Check sheet for the modelled part. Datum: model origin and axes. Units: mm. A direction names the side the tool comes from. Give positions to 0.01 mm unless a question says otherwise; leave off trailing zeros. Order: outer loops, then holes, each group sorted by start corner. A loop starts at its lowest first (then second) coordinate and runs counter-clockwise, first axis right, second up. Notation, with made-up numbers: (74, 64) -> (86, 64) arc R16 cw to (86, 86) -> close; hole circle Ø10 at (43.5, 65.25). An arc over 180 degrees is marked (long way). Write each question's results on one line, items separated by ' | '.
from build123d import *

# Parameters (mm, degrees)
SKETCH1_R           = 11.25
SKETCH1_R_2         = 11.05
BOSS_EXTRUDE1_DEPTH = 20
BOSS_EXTRUDE2_DEPTH = 2
SKETCH3_R           = 9.5
BOSS_EXTRUDE3_DEPTH = 18
SKETCH4_W           = 81.5
SKETCH4_H           = 10
CUT_EXTRUDE1_DEPTH  = 47
FILLET1_START       = -12
FILLET1_DEPTH       = 28
FILLET1_START_2     = -10.55574922
FILLET1_2_DEPTH     = 25.7
SKETCH5_W           = 47.5
SKETCH5_H           = 10
BOSS_EXTRUDE4_DEPTH = 20
FILLET2_R           = 5
SKETCH6_W           = 21.5
SKETCH6_H           = 25.70672576
CUT_EXTRUDE2_DEPTH  = 20
FILLET3_R           = 5
SKETCH7_R           = 2.25
CUT_EXTRUDE3_DEPTH  = 20
CUT_EXTRUDE4_DEPTH  = 4
FILLET4_R           = 5
FILLET5_R           = 5


with BuildPart() as part:
    # Sketch1 → Boss-Extrude1 (new body)
    with BuildSketch(Plane(origin=(0, 0, 0), x_dir=(1, 0, 0), z_dir=(0, 1, 0))):
        with BuildLine():
            Line((98.181049616, -15.14425078), (-23.318950384, -15.14425078))
            ThreePointArc((-23.318950384, -15.14425078), (-36.168950384, -2.29425078), (-23.318950384, 10.55574922))
            Line((-23.318950384, 10.55574922), (98.181049616, 10.55574922))
            ThreePointArc((98.181049616, 10.55574922), (111.031049616, -2.29425078), (98.181049616, -15.14425078))
        make_face()
        with Locations(Location((-23.318950384, -2.29425078, 0), (0, 0, 270))):
            Circle(SKETCH1_R, mode=Mode.SUBTRACT)
        with Locations(Location((98.181049616, -2.29425078, 0), (0, 0, 270))):
            Circle(SKETCH1_R_2, mode=Mode.SUBTRACT)
    extrude(amount=BOSS_EXTRUDE1_DEPTH)

    # Sketch2 → Boss-Extrude2 (add)
    with BuildSketch(Plane.XZ):
        with BuildLine():
            Line((-23.318950384, -10.55574922), (98.181049616, -10.55574922))
            ThreePointArc((98.181049616, -10.55574922), (111.031049616, 2.29425078), (98.181049616, 15.14425078))
            Line((98.181049616, 15.14425078), (-23.318950384, 15.14425078))
            ThreePointArc((-23.318950384, 15.14425078), (-36.168950384, 2.29425078), (-23.318950384, -10.55574922))
        make_face()
    extrude(amount=-BOSS_EXTRUDE2_DEPTH)

    # Sketch3 → Boss-Extrude3 (add)
    with BuildSketch(Plane(origin=(0, 2, 0), x_dir=(1, 0, 0), z_dir=(0, 1, 0))):
        with Locations(Location((-23.318950384, -2.29425078, 0), (0, 0, 90))):
            Circle(SKETCH3_R)
        with Locations(Location((98.181049616, -2.29425078, 0), (0, 0, 90))):
            Circle(SKETCH3_R)
    extrude(amount=BOSS_EXTRUDE3_DEPTH)

    # Sketch4 → Cut-Extrude1 (cut)
    with BuildSketch(Plane(origin=(0, 0, -10.55574922), x_dir=(-1, 0, 0), z_dir=(0, 0, -1))):
        with Locations((-37.431049616, 5)):
            Rectangle(SKETCH4_W, SKETCH4_H)
    extrude(amount=-CUT_EXTRUDE1_DEPTH, mode=Mode.SUBTRACT)

    # Fillet1: read off the stored shape, not the designer's step
    # Fillet1 outline → Fillet1 (cut)
    with BuildSketch(Plane.XY.offset(FILLET1_START)):
        with BuildLine():
            Line((-3.318950384, 0), (-3.318950384, 5))
            ThreePointArc((-3.318950384, 5), (-4.783416479, 1.464466094), (-8.318950384, 0))
            Line((-8.318950384, 0), (-3.318950384, 0))
        make_face()
        with BuildLine():
            ThreePointArc((83.181049616, 0), (79.64551571, 1.464466094), (78.181049616, 5))
            Line((78.181049616, 5), (78.181049616, 0))
            Line((78.181049616, 0), (83.181049616, 0))
        make_face()
    extrude(amount=FILLET1_DEPTH, mode=Mode.SUBTRACT)

    # Fillet1 2 outline → Fillet1 2 (add)
    with BuildSketch(Plane.XY.offset(FILLET1_START_2)):
        with BuildLine():
            Line((78.181049616, 10), (73.181049616, 10))
            ThreePointArc((73.181049616, 10), (76.716583521, 8.535533906), (78.181049616, 5))
            Line((78.181049616, 5), (78.181049616, 10))
        make_face()
        with BuildLine():
            ThreePointArc((-3.318950384, 5), (-1.85448429, 8.535533906), (1.681049616, 10))
            Line((1.681049616, 10), (-3.318950384, 10))
            Line((-3.318950384, 10), (-3.318950384, 5))
        make_face()
    extrude(amount=FILLET1_2_DEPTH)

    # Sketch5 → Boss-Extrude4 (add)
    with BuildSketch(Plane(origin=(0, 0, -10.55574922), x_dir=(-1, 0, 0), z_dir=(0, 0, -1))):
        with Locations((-37.431049616, 15)):
            Rectangle(SKETCH5_W, SKETCH5_H)
    extrude(amount=BOSS_EXTRUDE4_DEPTH)

    # Fillet2
    fillet2_edges = [part.edges().sort_by_distance(p)[0] for p in [
        (13.681049616, 15, -10.55574922),
        (61.181049616, 15, -10.55574922),
        (13.681049616, 15, -30.55574922),
        (61.181049616, 15, -30.55574922),
    ]]
    fillet(fillet2_edges, radius=FILLET2_R)

    # Sketch6 → Cut-Extrude2 (cut)
    with BuildSketch(Plane(origin=(0, 10, 0), x_dir=(-1, 0, 0), z_dir=(0, -1, 0))):
        with Locations((-37.431049616, -2.2908879)):
            Rectangle(SKETCH6_W, SKETCH6_H)
    extrude(amount=-CUT_EXTRUDE2_DEPTH, mode=Mode.SUBTRACT)

    # Fillet3
    fillet3_edges = [part.edges().sort_by_distance(p)[0] for p in [
        (26.681049616, 15, -10.56247498),
        (26.681049616, 15, 15.14425078),
        (48.181049616, 15, 15.14425078),
        (48.181049616, 15, -10.56247498),
    ]]
    fillet(fillet3_edges, radius=FILLET3_R)

    # Sketch7 → Cut-Extrude3 (cut)
    with BuildSketch(Plane(origin=(0, 10, 0), x_dir=(-1, 0, 0), z_dir=(0, -1, 0))):
        with Locations(Location((-27.431049616, 24.55574922, 0), (0, 0, 180))):
            Circle(SKETCH7_R)
        with Locations(Location((-47.431049616, 24.55574922, 0), (0, 0, 180))):
            Circle(SKETCH7_R)
    extrude(amount=-CUT_EXTRUDE3_DEPTH, mode=Mode.SUBTRACT)

    # Sketch8 → Cut-Extrude4 (cut)
    with BuildSketch(Plane(origin=(0, 20, 0), x_dir=(1, 0, 0), z_dir=(0, 1, 0))):
        Polygon((31.424828925, 23.936830678), (29.963938451, 27.705004288), (25.970159141, 28.32392283), (23.437270306, 25.174667762), (24.898160781, 21.406494152), (28.89194009, 20.78757561), align=None)
        Polygon((51.424828925, 23.936830678), (49.963938451, 27.705004288), (45.970159141, 28.32392283), (43.437270306, 25.174667762), (44.898160781, 21.406494152), (48.89194009, 20.78757561), align=None)
    extrude(amount=-CUT_EXTRUDE4_DEPTH, mode=Mode.SUBTRACT)

    # Fillet4
    fillet4_edges = [part.edges().sort_by_distance(p)[0] for p in [
        (-23.318950384, 20, 11.79425078),
    ]]
    fillet(fillet4_edges, radius=FILLET4_R)

    # Fillet5
    fillet5_edges = [part.edges().sort_by_distance(p)[0] for p in [
        (98.181049616, 20, 11.79425078),
    ]]
    fillet(fillet5_edges, radius=FILLET5_R)


solid = part.part
1. Section check A-A on y = 7.5. Record the cut outline in (x, z), then the cut area to 3 significant figures.
Verdict:
outline: circle Ø19 at (-23.32, 2.29); (-23.32, -10.56) -> (-2.65, -10.56) -> (-2.65, 15.14) -> (-23.32, 15.14) arc R12.85 ccw to start; (77.51, -10.56) -> (98.18, -10.56) arc R12.85 ccw to (98.18, 15.14) -> (77.51, 15.14) -> close; circle Ø19 at (98.18, 2.29); hole circle Ø22.5 at (-23.32, 2.29); hole circle Ø22.1 at (98.18, 2.29) | area: 1,370 mm^2
2. Mould release check, pull along Z, two halves, no side actions. Record for faces 4 (the flat face through (38, 15, -10.562)), 5 (the flat face through (38, 15, -30.556)), 6 (the cylindrical face through (29.577, 12.958, -23.88)), 7 (the flat face through (48.181, 15, 2)): +Z half, -Z half, draft (parallel to the pull), parting line (faces both ways), or undercut.
Verdict:
face 4: +Z half | face 5: -Z half | face 6: undercut | face 7: draft
3. Section check B-B on x = 80. Record the cut outline in (y, z).
Verdict:
outline: (1.14, -10.56) -> (20, -10.56) -> (20, 15.14) -> (1.14, 15.14) -> close
4. Access from +Z, -Z, +X, -X, +Y, -Y to the whole of each face (thin tool, end or side, straight path). Record for faces 1 (the cylindrical face through (25.177, 15.07, 13.718)), 2 (the cylindrical face through (49.577, 12.958, -23.88)), 3 (the flat face through (44.157, 18.028, -23.317)).
Verdict:
face 1: +Z, +Y, -Y | face 2: +Y, -Y | face 3: +Y
5. Gauge pin test, flat ends, axial feed: pin 1 Ø6 at (x, y) = (-4.5, 9) entering from -Z; pin 2 Ø6 at (x, z) = (38.5, -19) entering from -Y; pin 3 Ø5 at (y, z) = (14, -21) entering from +X. Record the tip position at first contact, or that the pin passes through.
Verdict:
pin 1: stops at z = -10.56 | pin 2: stops at y = 10 | pin 3: stops at x = 61.18
6. Material ranges on probe 1 along X at (y, z) = (7, 7); probe 2 along X at (y, z) = (13.5, -25); probe 3 along X at (y, z) = (2.25, 10.5), recorded low to high. Write a range as from..to.
Verdict:
probe 1: x = -35.28..-33.54, -31.57..-15.07, -13.1..-2.9, 77.76..88.18, 89.93..106.43, 108.18..110.14 | probe 2: x = 13.68..25.23, 29.64..45.23, 49.64..61.18 | probe 3: x = -33.21..-31.01, -28.11..-18.53, -15.62..-4.14, 79.01..90.78, 93.39..102.97, 105.58..108.07
7. Section check C-C on z = -12. Record the cut outline in (x, y), then the cut area to 3 significant figures.
Verdict:
outline: (12.2, 10) -> (62.67, 10) -> (62.67, 20) -> (12.2, 20) -> close | area: 505 mm^2
